from build123d import *

# Parameters (mm, degrees)
BOX001_W          = 32
BOX001_H          = 15
BOX001_DEPTH      = 2
CYLINDER005_R     = 3.5
CYLINDER005_DEPTH = 2
CYLINDER004_R     = 17
CYLINDER004_DEPTH = 2
CYLINDER003_R     = 1.5
CYLINDER003_DEPTH = 15
CYLINDER002_R     = 1.5
CYLINDER002_DEPTH = 15
CYLINDER001_R     = 1.5
CYLINDER001_DEPTH = 15
CYLINDER_R        = 1.5
CYLINDER_DEPTH    = 15
BOX_W             = 32
BOX_H             = 32
BOX_DEPTH         = 3


with BuildPart() as cube001:
    # Box001 → Box001 (new body)
    with BuildSketch(Plane(origin=(0, -13, 0), x_dir=(1, 0, 0), z_dir=(0, 0, 1))):
        with Locations((16, 7.5)):
            Rectangle(BOX001_W, BOX001_H)
    extrude(amount=BOX001_DEPTH)


with BuildPart() as cylinder005:
    # Cylinder005 → Cylinder005 (new body)
    with BuildSketch(Plane(origin=(16, -17.5, 0), x_dir=(1, 0, 0), z_dir=(0, 0, 1))):
        Circle(CYLINDER005_R)
    extrude(amount=CYLINDER005_DEPTH)


with BuildPart() as cut:
    # Cylinder004 → Cylinder004 (new body)
    with BuildSketch(Plane(origin=(16, -17.5, 0), x_dir=(1, 0, 0), z_dir=(0, 0, 1))):
        Circle(CYLINDER004_R)
    extrude(amount=CYLINDER004_DEPTH)

    # Cut: cut Cylinder005
    add(cylinder005.part, mode=Mode.SUBTRACT)


with BuildPart() as cylinder003:
    # Cylinder003 → Cylinder003 (new body)
    with BuildSketch(Plane(origin=(29.5, 29.5, 0), x_dir=(1, 0, 0), z_dir=(0, 0, 1))):
        Circle(CYLINDER003_R)
    extrude(amount=CYLINDER003_DEPTH)


with BuildPart() as cylinder002:
    # Cylinder002 → Cylinder002 (new body)
    with BuildSketch(Plane(origin=(2.5, 29.5, 0), x_dir=(1, 0, 0), z_dir=(0, 0, 1))):
        Circle(CYLINDER002_R)
    extrude(amount=CYLINDER002_DEPTH)


with BuildPart() as cylinder001:
    # Cylinder001 → Cylinder001 (new body)
    with BuildSketch(Plane(origin=(29.5, 2.5, 0), x_dir=(1, 0, 0), z_dir=(0, 0, 1))):
        Circle(CYLINDER001_R)
    extrude(amount=CYLINDER001_DEPTH)


with BuildPart() as cylinder:
    # Cylinder → Cylinder (new body)
    with BuildSketch(Plane(origin=(2.5, 2.5, 0), x_dir=(1, 0, 0), z_dir=(0, 0, 1))):
        Circle(CYLINDER_R)
    extrude(amount=CYLINDER_DEPTH)


with BuildPart() as fusion005:
    # Box → Box (new body)
    with BuildSketch(Plane.XY):
        with Locations((16, 16)):
            Rectangle(BOX_W, BOX_H)
    extrude(amount=BOX_DEPTH)

    # Fusion: union Cylinder
    add(cylinder.part)

    # Fusion001: union Cylinder001
    add(cylinder001.part)

    # Fusion002: union Cylinder002
    add(cylinder002.part)

    # Fusion003: union Cylinder003
    add(cylinder003.part)

    # Fusion004: union Cut
    add(cut.part)

    # Fusion005: union Cube001
    add(cube001.part)


solid = fusion005.part
Input: part model. Units: mm. Frame: model coordinates. A direction names the side the tool comes from. Coordinates: 2 decimals unless noted, no trailing zeros. Order: outer loops, then holes, each group sorted by start corner. A loop starts at its lowest first (then second) coordinate and runs counter-clockwise, first axis right, second up.
1. Ray query, line 1 along Y through (x, z) = (16, 0.7); line 2 along Y through (x, z) = (13, 2.25); line 3 along Z through (x, y) = (3, -22.5). Return the intervals inside material, ascending.
Checked values:
line 1: y = -34.5 to -21, -14 to 32
line 2: y = 0 to 32
line 3: z = 0 to 2
2. Contact query for flat-ended pins moving along their axis: P1, Ø1, axis at x = 23.5, y = -17.5, coming from the +Z side; P2, Ø1.5, axis at y = 16.5, z = 1, coming from the +X side; P3, Ø5, axis at x = 22, z = 4.5, coming from the +Y side; P4, Ø1, axis at x = 13.5, y = 7, coming from the +Z side. Output: stop coordinate, or through.
Checked values:
P1: stops at z = 2
P2: stops at x = 32
P3: stops at y = 32
P4: stops at z = 3
3. Access query for faces 1 (the flat face through (32, 10, 1)), 2 (the flat face through (16, 32, 1)), 3 (the cylindrical face through (2.305, 30.987, 8.916)), 4 (the flat face through (16, -13, 2)). Directions: +Z, -Z, +X, -X, +Y, -Y. A direction counts if a zero-diameter tool reaches every point of the face in a straight line with its end or side. Return the directions, or none.
Checked values:
face 1: +Z, -Z, +X, +Y
face 2: +Z, -Z, +X, -X, +Y
face 3: +Z
face 4: +Z, +X, -X, -Y
4. Cut plane D-D, the plane z = 5. Return loops of the section in (x, y), plus the area to 3 significant figures.
Checked values:
outline: circle Ø3 at (2.5, 2.5); circle Ø3 at (2.5, 29.5); circle Ø3 at (29.5, 2.5); circle Ø3 at (29.5, 29.5)
area: 28.3 mm2
5. Cut plane B-B, the plane y = -17.5. Return loops of the section in (x, z).
Checked values:
outline: (-1, 0) - (12.5, 0) - (12.5, 2) - (-1, 2) - close; (19.5, 0) - (33, 0) - (33, 2) - (19.5, 2) - close
6. Cut plane A-A, the plane x = 16. Return loops of the section in (y, z).
Checked values:
outline: (-34.5, 0) - (-21, 0) - (-21, 2) - (-34.5, 2) - close; (-14, 0) - (32, 0) - (32, 3) - (0, 3) - (0, 2) - (-14, 2) - close
7. Draft query along X for faces 5 (the cylindrical face through (15.544, -34.494, 0.986)), 6 (the flat face through (16, 16, 3)), 7 (the flat face through (0, 10, 1)), 8 (the flat face through (16, -1, 0)). Return one class per face: +X half, -X half, draft (parallel to the pull), parting line (faces both ways), or undercut.
Checked values:
face 5: parting line
face 6: undercut
face 7: -X half
face 8: draft
8. Cut plane C-C, the plane y = 2.5. Return loops of the section in (x, z), plus the area to 3 significant figures.
Checked values:
outline: (0, 0) - (32, 0) - (32, 3) - (31, 3) - (31, 15) - (28, 15) - (28, 3) - (4, 3) - (4, 15) - (1, 15) - (1, 3) - (0, 3) - close
area: 168 mm2
